Here's how the part is built. I have some questions about the finished solid (model axes, mm). Round coordinates to 2 decimals unless told otherwise and drop trailing zeros. Write each loop counter-clockwise with the first axis right and the second up, starting at its lowest first coordinate (ties: lowest second). Pieces come first, ordered by that corner, then holes. Notation, with made-up numbers: M 40,-30 L 74,-30 A28 ccw 74,0 Z; hole C 29.25,45.5 d2. An arc over 180 degrees is marked long. Use one line per item in the form item = value. Start each with the question number.
Q1. I need wall thicknesses on line 1 along X through (y, z) = (6.5, -52.5); line 2 along X through (y, z) = (6.5, -79); line 3 along Z through (x, y) = (37, 5.5). Which ranges of each line are inside material? Lowest first, please. Write a range as from..to.
Q2. I'm going to push flat-ended pins straight in: pin 1 Ø4 at (x, z) = (82.5, -52) entering from -Y; pin 2 Ø1 at (x, y) = (18.5, 1) entering from -Z; pin 3 Ø1.5 at (x, y) = (121, 3.5) entering from -Z. Where does each tip first touch, or does it pass through?
Q3. I want a section at A-A on z = -6.5. List the corners of the cut face in (x, y) for me.
Q4. I want a section at D-D on x = 145. List the corners of the cut face in (y, z) for me.
Q5. I want a section at B-B on x = 56.5. State how many separate pieces and enclosed holes the cut face has, and give its area (3 significant figures).
```python
from build123d import *

# Parameters (mm, degrees)
SKETCH1_W                = 165
SKETCH1_H                = 225
BOSS_EXTRUDE1_DEPTH      = 8
SKETCH2_W                = 40
SKETCH2_H                = 70
CUT_EXTRUDE1_DEPTH       = 280.130793715
CHAMFER1_SIZE            = 60
M6_CLEARANCE_HOLE1_D     = 6.4
M6_CLEARANCE_HOLE1_DEPTH = 8
M6_CLEARANCE_HOLE1_TIP   = 1.922753981
M5_CLEARANCE_HOLE1_D     = 5.3
M5_CLEARANCE_HOLE1_DEPTH = 8
M5_CLEARANCE_HOLE1_TIP   = 1.59228064
M5_CLEARANCE_HOLE2_D     = 5.3
M5_CLEARANCE_HOLE2_DEPTH = 8
M5_CLEARANCE_HOLE2_TIP   = 1.59228064


with BuildPart() as part:
    # Sketch1 → Boss-Extrude1 (new body)
    with BuildSketch(Plane(origin=(0, 0, 0), x_dir=(1, 0, 0), z_dir=(0, 1, 0))):
        with Locations((82.5, 112.5)):
            Rectangle(SKETCH1_W, SKETCH1_H)
    extrude(amount=BOSS_EXTRUDE1_DEPTH)

    # Sketch2 → Cut-Extrude1 (cut, through all)
    with BuildSketch(Plane.XZ):
        with Locations((20, -82.5)):
            Rectangle(SKETCH2_W, SKETCH2_H)
    extrude(amount=-CUT_EXTRUDE1_DEPTH, mode=Mode.SUBTRACT)

    # Chamfer1
    chamfer1_edges = [part.edges().sort_by_distance(p)[0] for p in [
        (0, 4, -225),
        (165, 4, -225),
    ]]
    chamfer(chamfer1_edges, length=CHAMFER1_SIZE)

    # M6 Clearance Hole1
    with Locations(Plane(origin=(0, 8, 0), x_dir=(1, 0, 0), z_dir=(0, 1, 0))):
        with Locations((82.5, 210)):
            Hole(M6_CLEARANCE_HOLE1_D / 2, depth=M6_CLEARANCE_HOLE1_DEPTH)
            with Locations((0, 0, -(M6_CLEARANCE_HOLE1_DEPTH + M6_CLEARANCE_HOLE1_TIP / 2))):  # 118° drill point
                Cone(0, M6_CLEARANCE_HOLE1_D / 2, M6_CLEARANCE_HOLE1_TIP, mode=Mode.SUBTRACT)

    # M5 Clearance Hole1
    with Locations(Plane(origin=(0, 8, 0), x_dir=(1, 0, 0), z_dir=(0, 1, 0))):
        with Locations((7.5, 158.5), (37.5, 158.5), (37.5, 126.5), (7.5, 126.5), (158.5, 102.5), (134.5, 102.5), (157.5, 126.5), (127.5, 126.5), (127.5, 158.5), (157.5, 158.5), (157.5, 6.5), (127.5, 6.5), (127.5, 38.5), (157.5, 38.5), (134.5, 62.5), (158.5, 62.5), (7.5, 38.5), (37.5, 38.5), (37.5, 6.5), (7.5, 6.5)):
            Hole(M5_CLEARANCE_HOLE1_D / 2, depth=M5_CLEARANCE_HOLE1_DEPTH)
            with Locations((0, 0, -(M5_CLEARANCE_HOLE1_DEPTH + M5_CLEARANCE_HOLE1_TIP / 2))):  # 118° drill point
                Cone(0, M5_CLEARANCE_HOLE1_D / 2, M5_CLEARANCE_HOLE1_TIP, mode=Mode.SUBTRACT)

    # M5 Clearance Hole2
    with Locations(Plane(origin=(0, 8, 0), x_dir=(1, 0, 0), z_dir=(0, 1, 0))):
        with Locations((56.5, 26), (82.5, 26), (108.5, 26), (82.5, 52), (108.5, 52), (82.5, 78), (108.5, 78), (82.5, 104), (108.5, 104), (82.5, 130), (108.5, 130), (82.5, 156), (108.5, 156), (82.5, 182), (108.5, 182), (56.5, 52), (56.5, 78), (56.5, 104), (56.5, 130), (56.5, 156), (56.5, 182)):
            Hole(M5_CLEARANCE_HOLE2_D / 2, depth=M5_CLEARANCE_HOLE2_DEPTH)
            with Locations((0, 0, -(M5_CLEARANCE_HOLE2_DEPTH + M5_CLEARANCE_HOLE2_TIP / 2))):  # 118° drill point
                Cone(0, M5_CLEARANCE_HOLE2_D / 2, M5_CLEARANCE_HOLE2_TIP, mode=Mode.SUBTRACT)


solid = part.part
```
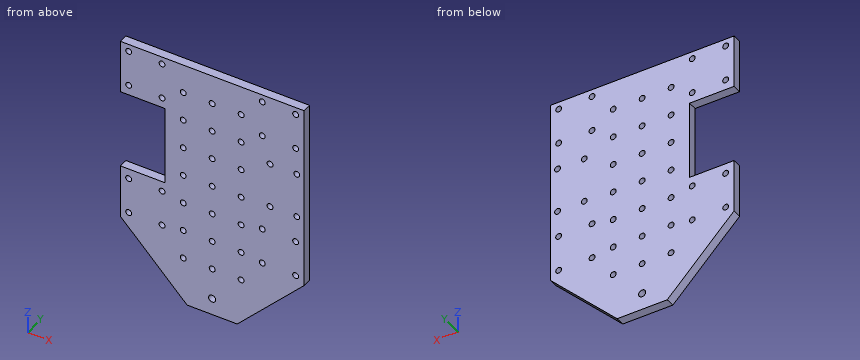
Reported:
q1.line_1 = 40..53.9, 59.1..79.9, 85.1..105.9, 111.1..165
q1.line_2 = 40..54.05, 58.95..80.05, 84.95..106.05, 110.95..165
q1.line_3 = -202..-161.1, -155.9..-129.1, -123.9..-117.5, -47.5..-41.1, -35.9..-9.1, -3.9..0
q2.pin_1 = through
q2.pin_2 = -184
q2.pin_3 = -209.75
q3.outline = M 0,0 L 4.85,0 L 4.85,8 L 0,8 Z; M 10.15,0 L 34.85,0 L 34.85,8 L 10.15,8 Z; M 40.15,0 L 124.85,0 L 124.85,8 L 40.15,8 Z; M 130.15,0 L 154.85,0 L 154.85,8 L 130.15,8 Z; M 160.15,0 L 165,0 L 165,8 L 160.15,8 Z
q4.outline = M 0,-185 L 8,-185 L 8,0 L 0,0 Z
q5.separate_pieces = 8
q5.enclosed_holes = 0
q5.area = 1,480 mm^2
